Build history of the part. All positions in model axes, mm. Round coordinates to 2 decimals unless told otherwise and drop trailing zeros. Write each loop counter-clockwise with the first axis right and the second up, starting at its lowest first coordinate (ties: lowest second). Pieces come first, ordered by that corner, then holes. Notation, with made-up numbers: M 31,87.25 L 38,87.25 A23 cw 38,100.25 Z; hole C 87,-16 d9. An arc over 180 degrees is marked long. Write item = value, one per line. Start each with the question number.
Q1. Band-saw the part on C-C on z = 3.65. Write the cut outline in (x, y).
Q2. Band-saw the part on A-A on y = 0. Write the cut outline in (x, z).
Q3. Band-saw the part on B-B on x = 95.25. Write the cut outline in (y, z), plus the area to 3 significant figures.
Q4. Probe L1, parallel to Y at x = -95.25, z = 1.4; L2, parallel to X at y = 1.25, z = 0.3. List the from-to ranges inside material, lowest first.
```python
from build123d import *

# Parameters (mm, degrees)
SKETCH1_W           = 203.2
SKETCH1_H           = 12.7
SKETCH1_R           = 2.38125
BOSS_EXTRUDE1_DEPTH = 4.7625


with BuildPart() as part:
    # Sketch1 → Boss-Extrude1 (new body)
    with BuildSketch(Plane.XY):
        Rectangle(SKETCH1_W, SKETCH1_H)
        with Locations(Location((95.25, 0, 0), (0, 0, 180))):
            Circle(SKETCH1_R, mode=Mode.SUBTRACT)
        with Locations(Location((44.45, 0, 0), (0, 0, 180))):
            Circle(SKETCH1_R, mode=Mode.SUBTRACT)
        with Locations(Location((-95.25, 0, 0), (0, 0, 180))):
            Circle(SKETCH1_R, mode=Mode.SUBTRACT)
    extrude(amount=BOSS_EXTRUDE1_DEPTH)


solid = part.part
```
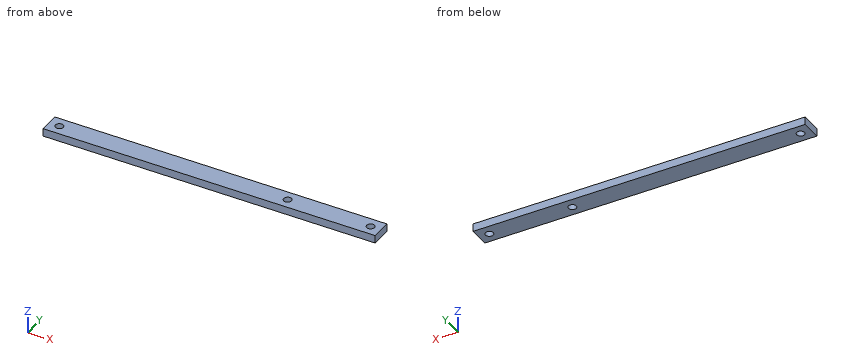
Conclusion:
q1.outline = M -101.6,-6.35 L 101.6,-6.35 L 101.6,6.35 L -101.6,6.35 Z; hole C -95.25,0 d4.76; hole C 44.45,0 d4.76; hole C 95.25,0 d4.76
q2.outline = M -101.6,0 L -97.63,0 L -97.63,4.76 L -101.6,4.76 Z; M -92.87,0 L 42.07,0 L 42.07,4.76 L -92.87,4.76 Z; M 46.83,0 L 92.87,0 L 92.87,4.76 L 46.83,4.76 Z; M 97.63,0 L 101.6,0 L 101.6,4.76 L 97.63,4.76 Z
q3.outline = M -6.35,0 L -2.38,0 L -2.38,4.76 L -6.35,4.76 Z; M 2.38,0 L 6.35,0 L 6.35,4.76 L 2.38,4.76 Z
q3.area = 37.8 mm^2
q4.L1 = -6.35 to -2.38, 2.38 to 6.35
q4.L2 = -101.6 to -97.28, -93.22 to 42.42, 46.48 to 93.22, 97.28 to 101.6
